Geometry check sheet. Reference: drawing and pictorial views, mm from the part's lowest x, y, z. Coordinates: 2 decimals unless noted, no trailing zeros. Loops run counter-clockwise (first coordinate to the right, second up) from the corner with the lowest first, then second, coordinate; pieces in that order, holes last. Notation, with made-up numbers: (27.25, 1) -> (56.25, 1) arc R17 cw to (56.25, 30) -> close; hole circle Ø5 at (42.25, 9.5). An arc over 180 degrees is marked (long way). Use one line per item in the form item = value.
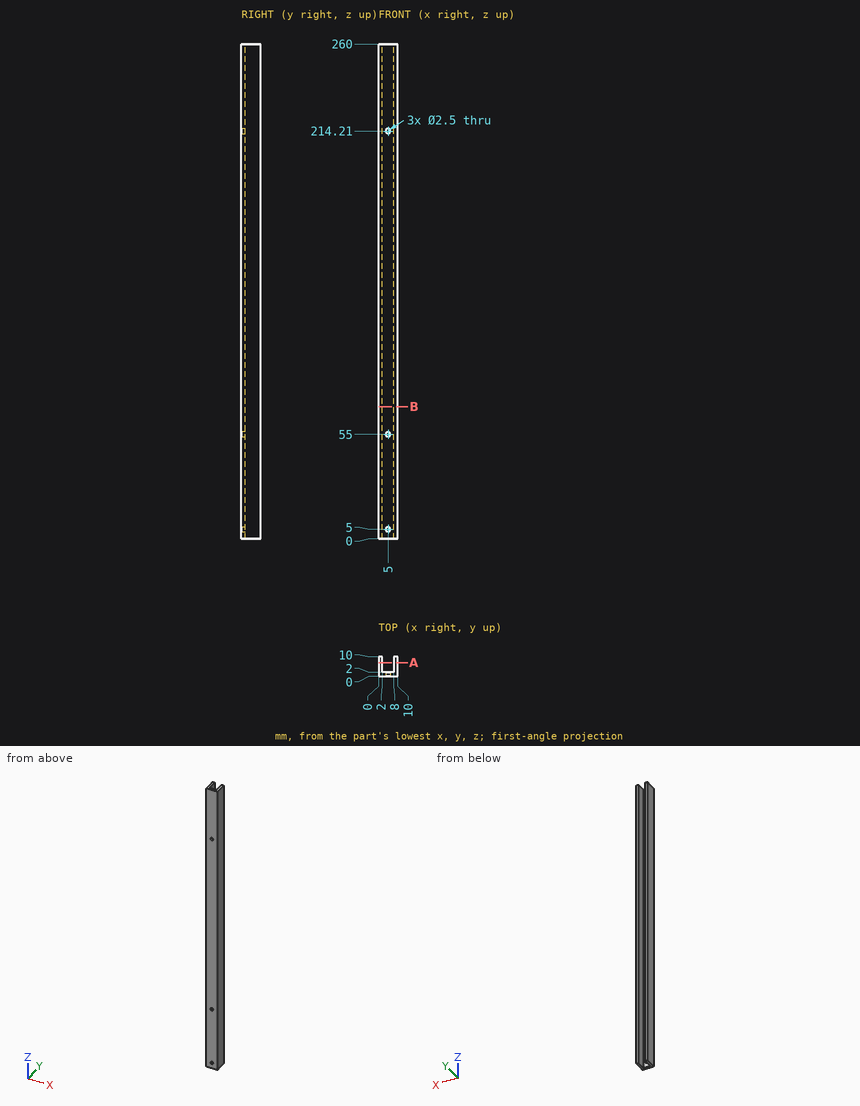
(1) Section check B-B, the plane z = 69.5. Record the boundary of the cut face in (x, y).
Established:
outline = (0, 0) -> (10, 0) -> (10, 10) -> (8, 10) -> (8, 2) -> (2, 2) -> (2, 10) -> (0, 10) -> close
(2) Section check A-A, the plane y = 7. Record the boundary of the cut face in (x, z), plus the area to 3 significant figures.
Established:
outline = (0, 0) -> (2, 0) -> (2, 260) -> (0, 260) -> close; (8, 0) -> (10, 0) -> (10, 260) -> (8, 260) -> close
area = 1,040 mm²
(3) Scan lines: line 1 along X through (y, z) = (8, 138); line 2 along X through (y, z) = (1.3, 5); line 3 along Y through (x, z) = (4, 185). Record each from-to range of solid material in increasing order.
Established:
line_1 = 0 to 2, 8 to 10
line_2 = 0 to 3.75, 6.25 to 10
line_3 = 0 to 2
(4) Go/stop test with flat-tipped pins: P1, Ø4, axis at x = 5, z = 214.21, coming from the -Y side; P2, Ø1, axis at x = 3.5, z = 54.5, coming from the +Y side. Record where each tip stops, or that it passes through.
Established:
P1 = 0
P2 = 2
